Can you work these out from the model? Positions are in its coordinate system, mm. Face numbers are marked on the shaded views. A direction names the side the tool comes from. Give positions to 0.01 mm unless a question says otherwise; leave off trailing zeros. Loops run counter-clockwise (first coordinate to the right, second up) from the corner with the lowest first, then second, coordinate; pieces in that order, holes last. Notation, with made-up numbers: (43.5, -7) - (88.5, -7) arc R19 cw to (88.5, 27) - close; hole circle Ø7 at (53, -5). An arc over 180 degrees is marked (long way). Answer as a JSON object with one key per item and string values. Group by question number.
Item 1: Will these pins go through, and if not, where does the flat tip stop? pin 1 (8 mm diameter, centred on x = 10.5, y = 3.5, fed in from +Z); pin 2 (3 mm diameter, centred on x = -2, y = -3.5, fed in from -Z); pin 3 (8.5 mm diameter, centred on x = 3, z = 1.5, fed in from +Y); pin 4 (1.5 mm diameter, centred on y = 14, z = 9, fed in from -X).
Item 2: Suppose I cut it at A-A on y = 4.5. Write out the boundary of the cut face in (x, z).
Item 3: Thinking about a two-plate mould opening in Z: for the marked faces 3 and 4, which applies, pulls with the +Z half, pulls with the -Z half, needs draft (parallel to the pull), parting line crosses it, or undercut?
Item 4: Which directions (+Z, -Z, +X, -X, +Y, -Y) give clear straight access to the entire face, cutting with the end or side of a thin tool? Please do the marked faces 1 and 2.
Item 5: Please list where these lines run through material, in increasing order: L1, parallel to Z at x = 0, y = 18.35; L2, parallel to Z at x = 0, y = 0.5; L3, parallel to Y at x = -3.75, z = -10.5.
from build123d import *

# Parameters (mm, degrees)
SKETCH2_R          = 13
SKETCH2_R_2        = 8.5
CUT_EXTRUDE1_DEPTH = 0.5


with BuildPart() as part:
    # Sketch1 → Revolve1 (revolve)
    with BuildSketch(Plane.XY):
        Polygon((8, -18.5), (8, 18.5), (13.5, 18.5), (14, 18), (14, 13.25), (13.5, 13.25), (13.5, 11.65), (14, 11.65), (14, -11.65), (13.5, -11.65), (13.5, -13.25), (14, -13.25), (14, -18), (13.5, -18.5), align=None)
    revolve(axis=Axis((0, 18.5, 0), (0, -1, 0)))

    # Sketch2 → Cut-Extrude1 (cut)
    with BuildSketch(Plane(origin=(0, 18.5, 0), x_dir=(1, 0, 0), z_dir=(0, 1, 0))):
        Circle(SKETCH2_R)
        Circle(SKETCH2_R_2, mode=Mode.SUBTRACT)
    cut_extrude1 = extrude(amount=-CUT_EXTRUDE1_DEPTH, mode=Mode.SUBTRACT)

    # Mirror1: Cut-Extrude1 across plane
    add(cut_extrude1.mirror(Plane.ZX), mode=Mode.SUBTRACT)


solid = part.part
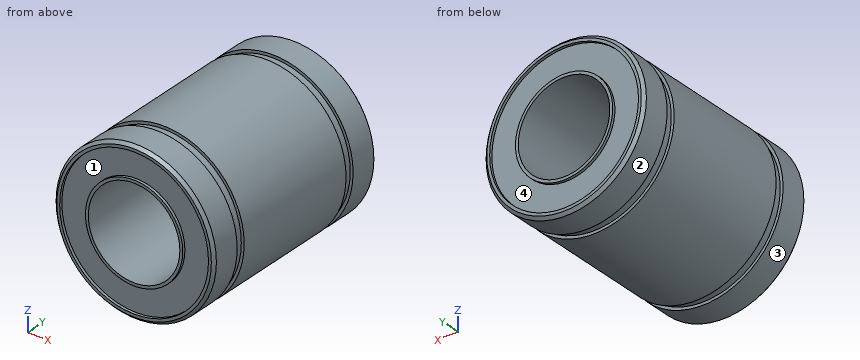
Worked out:
{
 "1": {"pin 1": "stops at z = 12.4", "pin 2": "stops at z = -13.99", "pin 3": "passes through", "pin 4": "stops at x = -11.31"},
 "2": {"outline": "circle Ø28 at (0, 0); hole circle Ø16 at (0, 0)"},
 "3": {"face 3": "parting line crosses it", "face 4": "undercut"},
 "4": {"face 1": "-Y", "face 2": "+Y, -Y"},
 "5": {"L1": "z = -13.65 to -13, -8.5 to -8, 8 to 8.5, 13 to 13.65", "L2": "z = -14 to -8, 8 to 14", "L3": "y = -18 to 18"}
}
